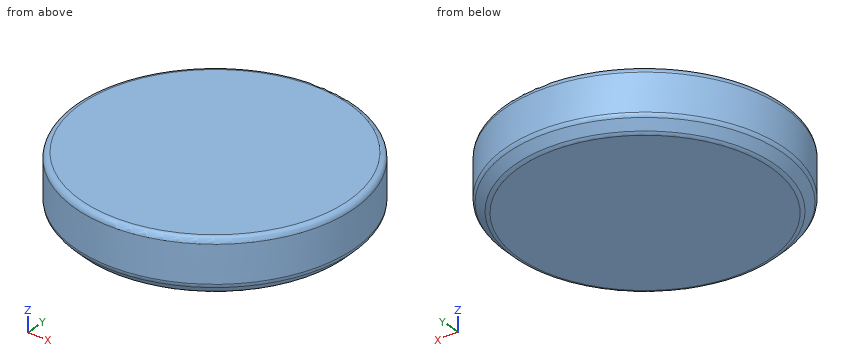
```python
from build123d import *

# Parameters (mm, degrees)
F0_R     = 12.25
F1_DEPTH = 5
F2_SIZE  = 1
F3_R     = 0.5


with BuildPart() as f1:
    # F0 (on Top) → F1 (new body)
    with BuildSketch(Plane.XY):
        Circle(F0_R)
    extrude(amount=F1_DEPTH)

    # F2
    f2_edges = [f1.edges().sort_by_distance(p)[0] for p in [
        (-12.25, 0, 0),
    ]]
    chamfer(f2_edges, length=F2_SIZE)

    # F3
    f3_edges = [f1.edges().sort_by_distance(p)[0] for p in [
        (-12.25, 0, 5),
        (-12.25, 0, 1),
        (-11.25, 0, 0),
    ]]
    fillet(f3_edges, radius=F3_R)


solid = f1.part
```
Source: CAD feature listing. Evaluate the final solid. Frame: model axes, mm. Coordinates: 2 decimals unless noted, no trailing zeros. Loops run counter-clockwise (first coordinate to the right, second up) from the corner with the lowest first, then second, coordinate; pieces in that order, holes last. Notation, with made-up numbers: (70, 40) -> (114, 40) arc R17 cw to (114, 58) -> close; hole circle Ø10 at (6, 20.25). An arc over 180 degrees is marked (long way). One line per item, written item: value. Start each with the question number.
Q1. Line query: line 1 along Y through (x, z) = (-6, 0.4); line 2 along Y through (x, z) = (-9.5, 1.65); line 3 along X through (y, z) = (2.25, 3.6). Output: solid intervals per line, ascending.
Q2. Section query A-A, the plane z = 4.1. Return the cut outline in (x, y).
Q3. Contact query for flat-ended pins moving along their axis: P1, Ø12, axis at x = -9.5, y = 4, coming from the -Z side; P2, Ø3, axis at x = 9.5, z = 2.5, coming from the -Y side; P3, Ø3, axis at x = 7, z = 2.5, coming from the +Y side. Output: stop coordinate, or through.
Results:
1. line 1: -9.99 to 9.99
1. line 2: -7.73 to 7.73
1. line 3: -12.04 to 12.04
2. outline: circle Ø24.5 at (0, 0)
3. P1: z = 0
3. P2: y = -9.28
3. P3: y = 10.95
